Geometry check sheet. Reference: the model listing, model coordinates, mm. Give positions to 0.01 mm unless a question says otherwise; leave off trailing zeros. Write each loop counter-clockwise with the first axis right and the second up, starting at its lowest first coordinate (ties: lowest second). Pieces come first, ordered by that corner, then holes. Notation, with made-up numbers: (9.5, -39.5) - (25.5, -39.5) arc R3 cw to (25.5, -35.5) - close; hole circle Ø4 at (-15.5, -5.75). An arc over 180 degrees is marked (long way). Use a Markdown table: item, result.
```python
from build123d import *

# Parameters (mm, degrees)
SKETCH1_W           = 70
SKETCH1_H           = 28
BOSS_EXTRUDE1_DEPTH = 8
SKETCH2_W           = 10
SKETCH2_H           = 10
CUT_EXTRUDE1_DEPTH  = 10
SKETCH3_R           = 2.15
CUT_EXTRUDE2_DEPTH  = 46.530209751
SKETCH5_W           = 16.977623655
SKETCH5_H           = 6.5
CUT_EXTRUDE4_DEPTH  = 39.535697736
SKETCH7_R           = 1.65
CUT_EXTRUDE5_DEPTH  = 10


# Read off the part's stored shape, not the designer's step: Cut-Revolve1
with BuildPart() as part:
    # Sketch1 → Boss-Extrude1 (new body)
    with BuildSketch(Plane(origin=(0, 0, 0), x_dir=(1, 0, 0), z_dir=(0, 1, 0))):
        Rectangle(SKETCH1_W, SKETCH1_H)
    extrude(amount=BOSS_EXTRUDE1_DEPTH)

    # Sketch2 → Cut-Extrude1 (cut)
    with BuildSketch(Plane(origin=(0, 8, 0), x_dir=(1, 0, 0), z_dir=(0, 1, 0))):
        with Locations((30, 0)):
            Rectangle(SKETCH2_W, SKETCH2_H)
    extrude(amount=-CUT_EXTRUDE1_DEPTH, mode=Mode.SUBTRACT)

    # Sketch3 → Cut-Extrude2 (cut, through all)
    with BuildSketch(Plane.XY.offset(14)):
        with Locations((31, 4)):
            Circle(SKETCH3_R)
    extrude(amount=-CUT_EXTRUDE2_DEPTH, mode=Mode.SUBTRACT)

    # Sketch5 → Cut-Extrude4 (cut, through all)
    with BuildSketch(Plane(origin=(0, 8, 0), x_dir=(1, 0, 0), z_dir=(0, 1, 0))):
        with Locations((-26.511188172, 10.75)):
            Rectangle(SKETCH5_W, SKETCH5_H)
        Polygon((-18.022376345, 14), (-18.022376345, 7.5), (1.977623655, 14), align=None)
        Polygon((1.977623655, -14), (-18.022376345, -7.5), (-18.022376345, -14), align=None)
        with Locations((-26.511188172, -10.75)):
            Rectangle(SKETCH5_W, SKETCH5_H)
    extrude(amount=-CUT_EXTRUDE4_DEPTH, mode=Mode.SUBTRACT)

    # Cut-Revolve1 outline → Cut-Revolve1 (revolve, cut)
    with BuildSketch(Plane(origin=(0, 4, 0), x_dir=(0, 1, 0), z_dir=(0, 0, -1))):
        with BuildLine():
            Line((0, -35), (8.5, -35))
            Line((8.5, -35), (8.5, -22.5))
            Line((8.5, -22.5), (14.560219779, -22.5))
            Line((14.560219779, -22.5), (14.560219779, 35))
            Line((14.560219779, 35), (0, 35))
            Line((0, 35), (0, -22.5))
            ThreePointArc((0, -22.5), (5, -27.5), (0, -32.5))
            Line((0, -32.5), (0, -35))
        make_face()
    revolve(axis=Axis((0, 4, 0), (1, 0, 0)), mode=Mode.SUBTRACT)

    # Sketch7 → Cut-Extrude5 (cut)
    with BuildSketch(Plane.XZ):
        with Locations(Location((-27.5, 0, 0), (0, 0, 270))):
            Circle(SKETCH7_R)
    extrude(amount=-CUT_EXTRUDE5_DEPTH, mode=Mode.SUBTRACT)


solid = part.part
```
1) Mould release check, pull along X, two halves, no side actions. Record for faces 1 (the flat face through (-26, 0, 1)), 2 (the cylindrical face through (-25.864, 3.944, 0.215)): pulls with the +X half, pulls with the -X half, needs draft (parallel to the pull), parting line crosses it, or undercut.
Working result:
| item | result |
|---|---|
| face 1 | needs draft |
| face 2 | undercut |
2) Section check D-D on x = -31.5. Record the boundary of the cut face in (y, z), then the cut area to 3 significant figures.
Working result:
| item | result |
|---|---|
| outline | circle Ø6 at (4, 0) |
| area | 28.3 mm² |
3) Section check A-A on z = 0. Record the boundary of the cut face in (x, y), then the cut area to 3 significant figures.
Working result:
| item | result |
|---|---|
| outline | (-30.5, 0) - (-29.15, 0) - (-29.15, 8) - (-30.5, 8) arc R5 ccw to start; (-25.85, 0) - (-24.5, 0) arc R5 ccw to (-24.5, 8) - (-25.85, 8) - close |
| area | 44.0 mm² |
4) Material ranges on L1, parallel to X at y = 5, z = 0; L2, parallel to X at y = 2.5, z = 0.25; L3, parallel to Y at x = -25.25, z = -2, recorded low to high. Write a range as from..to.
Working result:
| item | result |
|---|---|
| L1 | x = -32.4..-29.15, -25.85..-22.6 |
| L2 | x = -32.26..-29.13, -25.87..-22.74 |
| L3 | y = 0.01..7.99 |
5) Section check B-B on x = -27.5. Record the boundary of the cut face in (y, z).
Working result:
| item | result |
|---|---|
| outline | (0, -3) arc R5 ccw to (8, -3) - (8, -1.65) - (0, -1.65) - close; (0, 1.65) - (8, 1.65) - (8, 3) arc R5 ccw to (0, 3) - close |
6) Depth check by flat-ended pin: P1, Ø2, axis at y = 7, z = 1, coming from the -X side; P2, Ø3, axis at y = 3, z = 4, coming from the +X side; P3, Ø1, axis at x = -25, y = 7, coming from the +Z side. Enter the tip coordinate at first touch or a pass-through.
Working result:
| item | result |
|---|---|
| P1 | stops at x = -32.01 |
| P2 | stops at x = -23.24 |
| P3 | stops at z = 3.66 |
7) Section check C-C on y = 3.75. Record the boundary of the cut face in (x, z), then the cut area to 3 significant figures.
Working result:
| item | result |
|---|---|
| outline | circle Ø9.99 at (-27.5, 0); hole circle Ø3.3 at (-27.5, 0) |
| area | 69.8 mm² |
